Verification items for the finished model (mm, model axes). Face numbers are marked on the shaded views. A direction names the side the tool comes from. Give positions to 0.01 mm unless a question says otherwise; leave off trailing zeros. Write each loop counter-clockwise with the first axis right and the second up, starting at its lowest first coordinate (ties: lowest second). Pieces come first, ordered by that corner, then holes. Notation, with made-up numbers: (-21.5, 10.25) -> (4.5, 10.25) arc R14 ccw to (4.5, 24.25) -> close; hole circle Ø8 at (64.5, -1). An arc over 180 degrees is marked (long way). Answer as CSV lines item,"result".
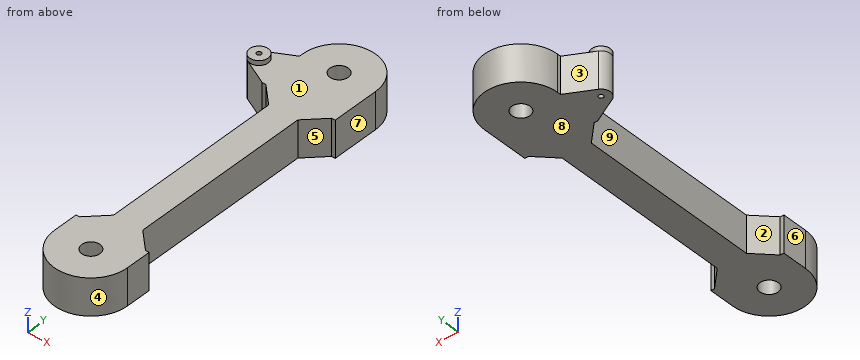
```python
from build123d import *

# Parameters (mm, degrees)
BOSS_EXTRUDE1_DEPTH     = 10
SKETCH2_R               = 2.5
CUT_EXTRUDE1_DEPTH      = 11
BOSS_EXTRUDE2_DEPTH     = 10
SKETCH4_R               = 0.635
CUT_EXTRUDE2_DEPTH      = 11
SKETCH5_R               = 2.54
SKETCH5_R_2             = 0.635
BOSS_EXTRUDE3_DEPTH     = 1.27
SKETCH6_W               = 6
SKETCH6_H               = 60
CUT_EXTRUDE3_DEPTH      = 2.27
CUT_EXTRUDE3_DEPTH_BACK = 11
CHAMFER1_SIZE           = 5


with BuildPart() as part:
    # Sketch1 → Boss-Extrude1 (new body)
    with BuildSketch(Plane.XY):
        with BuildLine():
            Line((-10, 80), (-10, 0))
            ThreePointArc((-10, 0), (0, -10), (10, 0))
            Line((10, 0), (10, 80))
            ThreePointArc((10, 80), (0, 90), (-10, 80))
        make_face()
    extrude(amount=BOSS_EXTRUDE1_DEPTH)

    # Sketch2 → Cut-Extrude1 (cut, through all)
    with BuildSketch(Plane.XY.offset(10)):
        Circle(SKETCH2_R)
        with Locations((0, 80)):
            Circle(SKETCH2_R)
    extrude(amount=-CUT_EXTRUDE1_DEPTH, mode=Mode.SUBTRACT)

    # Sketch3 → Boss-Extrude2 (add)
    with BuildSketch(Plane.XY.offset(10)):
        with BuildLine():
            Line((-10, 79), (-17.176061622, 75.251328288))
            ThreePointArc((-17.176061622, 75.251328288), (-18.54, 73), (-17.176061622, 70.748671712))
            Line((-17.176061622, 70.748671712), (-10, 67))
            Line((-10, 67), (-10, 79))
        make_face()
    extrude(amount=-BOSS_EXTRUDE2_DEPTH)

    # Sketch4 → Cut-Extrude2 (cut, through all)
    with BuildSketch(Plane.XY.offset(10)):
        with Locations((-16, 73)):
            Circle(SKETCH4_R)
    extrude(amount=-CUT_EXTRUDE2_DEPTH, mode=Mode.SUBTRACT)

    # Sketch5 → Boss-Extrude3 (add)
    with BuildSketch(Plane.XY.offset(10)):
        with Locations((-16, 73)):
            Circle(SKETCH5_R)
        with Locations((-16, 73)):
            Circle(SKETCH5_R_2, mode=Mode.SUBTRACT)
    extrude(amount=BOSS_EXTRUDE3_DEPTH)

    # Sketch6 → Cut-Extrude3 (cut, two sides)
    with BuildSketch(Plane.XY.offset(10)) as cut_extrude3_sk:
        with Locations((-7, 37)):
            Rectangle(SKETCH6_W, SKETCH6_H)
        with Locations((7, 37)):
            Rectangle(SKETCH6_W, SKETCH6_H)
    extrude(amount=CUT_EXTRUDE3_DEPTH, mode=Mode.SUBTRACT)
    extrude(cut_extrude3_sk.sketch, amount=-CUT_EXTRUDE3_DEPTH_BACK, mode=Mode.SUBTRACT)

    # Chamfer1
    chamfer1_edges = [part.edges().sort_by_distance(p)[0] for p in [
        (-4, 67, 5),
        (-4, 7, 5),
        (4, 7, 5),
        (4, 67, 5),
    ]]
    chamfer(chamfer1_edges, length=CHAMFER1_SIZE)


solid = part.part
```
1) Depth check by flat-ended pin: pin 1 (1 mm diameter, centred on x = -16, y = 73, fed in from +Z); pin 2 (0.5 mm diameter, centred on x = -9.5, z = 6, fed in from -Y); pin 3 (8 mm diameter, centred on x = -1, y = 62.5, fed in from +Z); pin 4 (0.8 mm diameter, centred on y = 79.5, z = 3, fed in from -X). Enter the tip coordinate at first touch or a pass-through.
Reported:
pin 1,"through"
pin 2,"y = -3.8"
pin 3,"z = 10"
pin 4,"x = -10"
2) Section check A-A (x = 0). Record the boundary of the cut face in (y, z).
Reported:
outline,"(-10, 0) -> (-2.5, 0) -> (-2.5, 10) -> (-10, 10) -> close; (2.5, 0) -> (77.5, 0) -> (77.5, 10) -> (2.5, 10) -> close; (82.5, 0) -> (90, 0) -> (90, 10) -> (82.5, 10) -> close"
3) Section check C-C (z = 6.75). Record the boundary of the cut face in (x, y) (3 decimals), and give its area (3 significant figures).
Reported:
outline,"(-17.176, 70.749) -> (-10, 67) -> (-9, 67) -> (-4, 62) -> (-4, 12) -> (-9, 7) -> (-10, 7) -> (-10, 0) arc R10 ccw to (10, 0) -> (10, 7) -> (9, 7) -> (4, 12) -> (4, 62) -> (9, 67) -> (10, 67) -> (10, 80) arc R10 ccw to (-10, 80) -> (-10, 79) -> (-17.176, 75.251) arc R2.54 ccw to start; hole circle Ø1.27 at (-16, 73); hole circle Ø5 at (0, 0); hole circle Ø5 at (0, 80)"
area,"1,270 mm²"
4) Scan lines: line 1 along Y through (x, z) = (0, 7.25); line 2 along Z through (x, y) = (-10.25, 77.5); line 3 along X through (y, z) = (73, 10.5) (3 decimals). Record each from-to range of solid material in increasing order.
Reported:
line 1,"-10 to -2.5, 2.5 to 77.5, 82.5 to 90"
line 2,"0 to 10"
line 3,"-18.54 to -16.635, -15.365 to -13.46"
5) Section check B-B (x = -8). Record the boundary of the cut face in (y, z), and give its area (3 significant figures).
Reported:
outline,"(-6, 0) -> (8, 0) -> (8, 10) -> (-6, 10) -> close; (66, 0) -> (86, 0) -> (86, 10) -> (66, 10) -> close"
area,"340 mm²"
6) Section check D-D (y = 28.5). Record the boundary of the cut face in (x, z), and give its area (3 significant figures).
Reported:
outline,"(-4, 0) -> (4, 0) -> (4, 10) -> (-4, 10) -> close"
area,"80.0 mm²"
7) Tool access check on the marked faces 5, 6, 7, 8 and 9. Record the directions out of +Z, -Z, +X, -X, +Y, -Y that give a thin tool (end or side, any length) a straight path to the whole face; none if there is none.
Reported:
face 5,"+Z, -Z, +X"
face 6,"+Z, -Z, -X, -Y"
face 7,"+Z, -Z, +X, +Y, -Y"
face 8,"-Z, +X, -X, +Y, -Y"
face 9,"+Z, -Z, -X"
8) Draft check along Y on the marked faces 1, 2, 3 and 4. Enter one of: +Y half, -Y half, draft (parallel to the pull), parting line (faces both ways), or undercut.
Reported:
face 1,"draft"
face 2,"undercut"
face 3,"+Y half"
face 4,"-Y half"
